Study the drawing (mm; zero at the part's minimum x, y, z) and answer. A direction names the side the tool comes from. Give positions to 0.01 mm unless a question says otherwise; leave off trailing zeros. Loops run counter-clockwise (first coordinate to the right, second up) from the corner with the lowest first, then second, coordinate; pieces in that order, holes last. Notation, with made-up numbers: M 65.5,-26.75 L 82.5,-26.75 A28 cw 82.5,6.25 Z; hole C -37.5,30 d1. An arc over 180 degrees is marked long. Return JSON: item names as keys, results as strings.
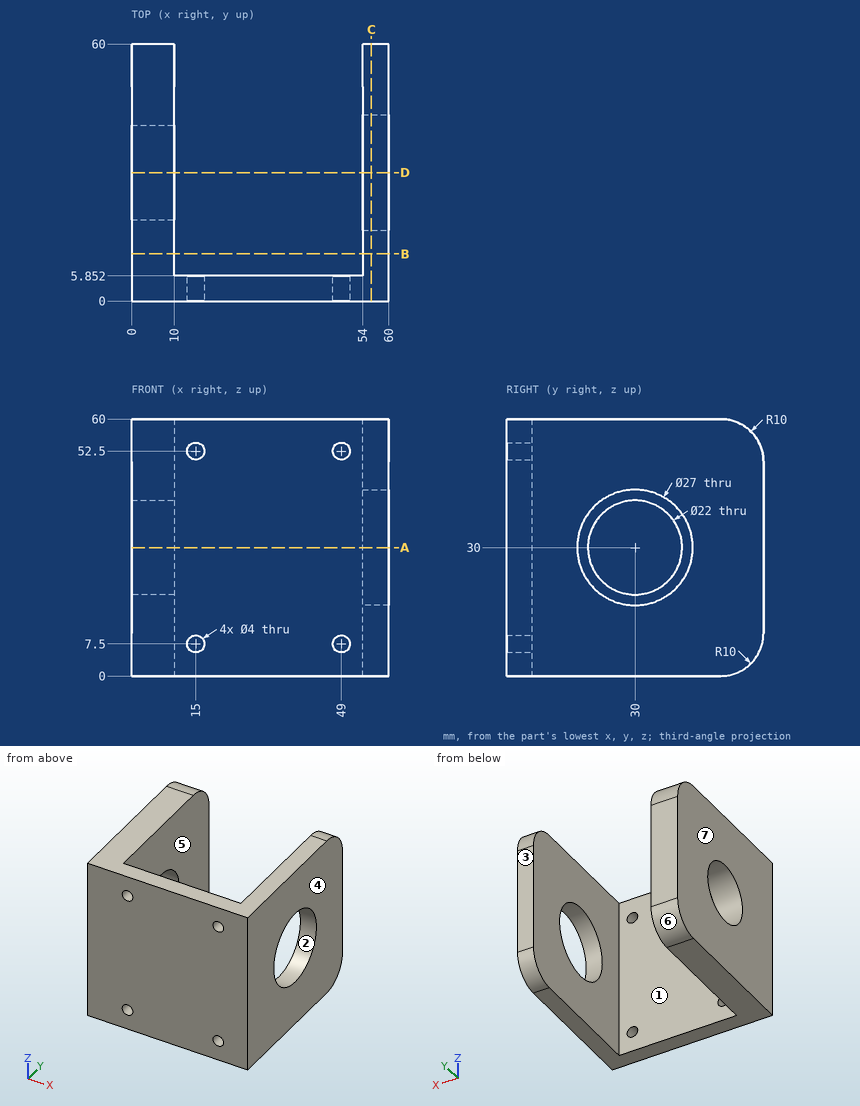
(1) The part is cut by section D-D (y = 30). Determine the outline of the cut face in (x, z).
Values follow:
{"outline": "M 0,0 L 10,0 L 10,19 L 0,19 Z; M 0,41 L 10,41 L 10,60 L 0,60 Z; M 54,0 L 60,0 L 60,16.5 L 54,16.5 Z; M 54,43.5 L 60,43.5 L 60,60 L 54,60 Z"}
(2) Given pin 1 (4 mm diameter, centred on x = 17.5, z = 15.5, fed in from +Y), flat-ended and moving along its own axis, determine where the tip first touches the part or whether it passes through.
Values follow:
{"pin 1": "y = 5.85"}
(3) Determine the mould class of the marked faces 4, 5, 6 and 7 for opening direction X: released by +X, released by -X, zero draft, split by the parting line, or undercut.
Values follow:
{"face 4": "released by +X", "face 5": "undercut", "face 6": "zero draft", "face 7": "released by -X"}
(4) The part is cut by section A-A (z = 30). Determine the outline of the cut face in (x, y), and give its area (4 significant figures).
Values follow:
{"outline": "M 0,0 L 60,0 L 60,16.5 L 54,16.5 L 54,5.85 L 10,5.85 L 10,19 L 0,19 Z; M 0,41 L 10,41 L 10,60 L 0,60 Z; M 54,43.5 L 60,43.5 L 60,60 L 54,60 Z", "area": "835.5 mm²"}
(5) A tool of negligible diameter and unlimited length cuts with its end or side. For the marked faces 1, 2 and 3, from which of +Z, -Z, +X, -X, +Y, -Y can it reach the whole face along a straight path? Write none if from no direction.
Values follow:
{"face 1": "+Z, -Z, +Y", "face 2": "+X", "face 3": "+Z, -Z, +X, -X, +Y"}
(6) The part is cut by section B-B (y = 11). Determine the outline of the cut face in (x, z), and give its area (3 significant figures).
Values follow:
{"outline": "M 0,0 L 10,0 L 10,60 L 0,60 Z; M 54,0 L 60,0 L 60,60 L 54,60 Z", "area": "960 mm²"}
(7) The part is cut by section C-C (x = 56). Determine the outline of the cut face in (y, z).
Values follow:
{"outline": "M 0,0 L 50,0 A10 ccw 60,10 L 60,50 A10 ccw 50,60 L 0,60 Z; hole C 30,30 d27"}
(8) Straight lines are drawn through the part: line 1 along Z through (x, y) = (15, 4.6); line 2 along X through (y, z) = (23, 47.5); line 3 along Y through (x, z) = (58.05, 30). For each, find the intervals that lie inside material, in ascending order.
Values follow:
{"line 1": "0 to 5.5, 9.5 to 50.5, 54.5 to 60", "line 2": "0 to 10, 54 to 60", "line 3": "0 to 16.5, 43.5 to 60"}
